Design review of the part built by this model. Coordinates are the model's own, in mm. Face numbers are marked on the shaded views. Coordinates: 2 decimals unless noted, no trailing zeros. Order: outer loops, then holes, each group sorted by start corner. A loop starts at its lowest first (then second) coordinate and runs counter-clockwise, first axis right, second up. Notation, with made-up numbers: (36, 46) -> (93, 46) arc R9 ccw to (93, 59) -> close; hole circle Ø5 at (54, 84.5). An arc over 180 degrees is marked (long way). Write item = value, one per line.
```python
from build123d import *

# Parameters (mm, degrees)
SKETCH_1_R               = 11
SKETCH_1_R_2             = 3
SKETCH_1_R_3             = 1.5
EXTRUDE_1_DEPTH          = 10
CUT_EXTRUDE_1_REACH      = 20.493
CUT_EXTRUDE_1_END_RADIUS = 11
SKETCH_2_R               = 1.5
CUT_EXTRUDE_2_REACH      = 20.493
CUT_EXTRUDE_2_END_RADIUS = 11
SKETCH_3_R               = 1.5


with BuildPart() as part:
    # ｽｹｯﾁ1 → ﾎﾞｽ - 押し出し1 (new body)
    with BuildSketch(Plane.XY):
        Circle(SKETCH_1_R)
        Circle(SKETCH_1_R_2, mode=Mode.SUBTRACT)
        with Locations((-7.5, 0)):
            Circle(SKETCH_1_R_3, mode=Mode.SUBTRACT)
        with Locations((7.5, 0)):
            Circle(SKETCH_1_R_3, mode=Mode.SUBTRACT)
        with Locations((0, 7.5)):
            Circle(SKETCH_1_R_3, mode=Mode.SUBTRACT)
        with Locations((0, -7.5)):
            Circle(SKETCH_1_R_3, mode=Mode.SUBTRACT)
    extrude(amount=EXTRUDE_1_DEPTH)

    # ｶｯﾄ - 押し出し1: up to this cylinder (the profile starts inside it)
    cut_extrude_1_end = Plane(origin=(0, 0, 5), z_dir=(0, 0, -1)) * Cylinder(CUT_EXTRUDE_1_END_RADIUS, 63.986, mode=Mode.PRIVATE)
    # ｽｹｯﾁ2 → ｶｯﾄ - 押し出し1 (cut, up to the surface)
    with BuildSketch(Plane(origin=(0, 0, 0), x_dir=(0.7071067811865477, -0.7071067811865475, 0), z_dir=(0.7071067811865475, 0.7071067811865477, 0)), mode=Mode.PRIVATE) as cut_extrude_1_sk1:
        with Locations((0, -5)):
            Circle(SKETCH_2_R)
    cut_extrude_1_tool1 = extrude(cut_extrude_1_sk1.sketch, amount=CUT_EXTRUDE_1_REACH, mode=Mode.PRIVATE) & cut_extrude_1_end
    add(cut_extrude_1_tool1.solids().sort_by_distance((0, 0, 5))[0], mode=Mode.SUBTRACT)

    # ｶｯﾄ - 押し出し2: up to this cylinder (the profile starts inside it)
    cut_extrude_2_end = Plane(origin=(0, 0, 5), z_dir=(0, 0, -1)) * Cylinder(CUT_EXTRUDE_2_END_RADIUS, 63.986, mode=Mode.PRIVATE)
    # ｽｹｯﾁ3 → ｶｯﾄ - 押し出し2 (cut, up to the surface)
    with BuildSketch(Plane(origin=(0, 0, 0), x_dir=(0.7071067811865477, 0.7071067811865475, 0), z_dir=(-0.7071067811865475, 0.7071067811865477, 0)), mode=Mode.PRIVATE) as cut_extrude_2_sk1:
        with Locations(Location((0, -5, 0), (0, 0, 180))):
            Circle(SKETCH_3_R)
    cut_extrude_2_tool1 = extrude(cut_extrude_2_sk1.sketch, amount=-CUT_EXTRUDE_2_REACH, mode=Mode.PRIVATE) & cut_extrude_2_end
    add(cut_extrude_2_tool1.solids().sort_by_distance((0, 0, 5))[0], mode=Mode.SUBTRACT)


solid = part.part
```
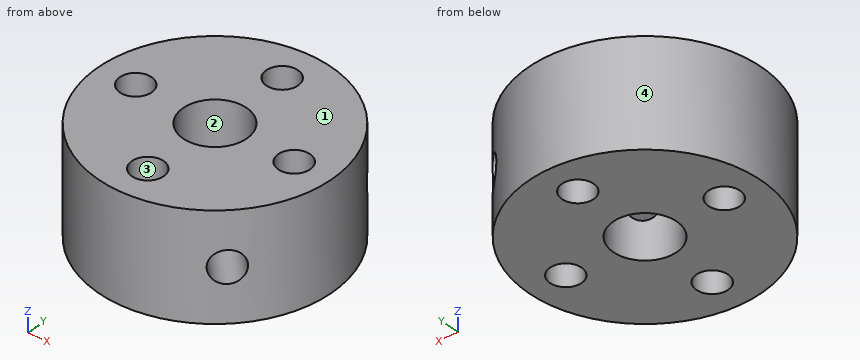
(1) We need section B-B (z = 2.5). Write out the cut boundary in (x, y).
Report:
outline = circle Ø22 at (0, 0); hole circle Ø3 at (-7.5, 0); hole circle Ø6 at (0, 0); hole circle Ø3 at (0, -7.5); hole circle Ø3 at (0, 7.5); hole circle Ø3 at (7.5, 0)
(2) We need section A-A (y = 0). Write out the cut boundary in (x, z).
Report:
outline = (-11, 0) -> (-9, 0) -> (-9, 10) -> (-11, 10) -> close; (-6, 0) -> (-3, 0) -> (-3, 10) -> (-6, 10) -> close; (3, 0) -> (6, 0) -> (6, 10) -> (3, 10) -> close; (9, 0) -> (11, 0) -> (11, 10) -> (9, 10) -> close
(3) We need section C-C (z = 5.5). Write out the cut boundary in (x, y).
Report:
outline = (0.87, -2.87) arc R3 cw (long way) to (0.87, 2.87) -> (6.71, 8.71) arc R11 ccw (long way) to (6.71, -8.71) -> close; (2.87, -0.87) -> (8.71, -6.71) arc R11 ccw to (8.71, 6.71) -> (2.87, 0.87) arc R3 cw to start; hole circle Ø3 at (-7.5, 0); hole circle Ø3 at (0, -7.5); hole circle Ø3 at (0, 7.5); hole circle Ø3 at (7.5, 0)
(4) For L1, parallel to Y at x = 0, z = 5.5; L2, parallel to X at y = 1, z = 5.25; L3, parallel to Z at x = 7.5, y = 7.5, list the stretches that pass through material, from the lowest coordinate up.
Report:
L1 = -11 to -9, -6 to -3, 3 to 6, 9 to 11
L2 = -10.95 to -8.62, -6.38 to -2.83, 3.09 to 6.38, 8.62 to 10.95
L3 = 0 to 3.5, 6.5 to 10
(5) The part is to be moulded in two halves that separate along X. For the marked faces 1, 2, 3 and 4, say which applies: released by +X, released by -X, zero draft, split by the parting line, or undercut.
Report:
face_1 = zero draft
face_2 = undercut
face_3 = undercut
face_4 = split by the parting line
(6) We need section D-D (x = -7.5). Write out the cut boundary in (y, z).
Report:
outline = (-8.05, 0) -> (-1.5, 0) -> (-1.5, 10) -> (-8.05, 10) -> close; (1.5, 0) -> (8.05, 0) -> (8.05, 10) -> (1.5, 10) -> close
(7) Insertion check: pin 1 (5 mm diameter, centred on x = 0, y = 0, fed in from +Z); pin 2 (1.5 mm diameter, centred on x = -6, z = 2, fed in from -Y); pin 3 (1.5 mm diameter, centred on y = 1.5, z = 1.5, fed in from -X); pin 4 (1 mm diameter, centred on x = 2.5, z = 8, fed in from +Y). Each pin has a flat end and moves straight along its axis. Give the tip position at first contact, or say it passes through.
Report:
pin_1 = through
pin_2 = -9.67
pin_3 = -10.97
pin_4 = 10.82
